Model file for the job. Use its own axes, mm. Coordinates: 2 decimals unless noted, no trailing zeros. Loops run counter-clockwise (first coordinate to the right, second up) from the corner with the lowest first, then second, coordinate; pieces in that order, holes last. Notation, with made-up numbers: (23.25, 24) -> (40.25, 24) arc R9 cw to (40.25, 34) -> close; hole circle Ø2 at (69.25, -17.75). An arc over 180 degrees is marked (long way). Use one line per item in the form item = value.
```python
from build123d import *

# Parameters (mm, degrees)
F0_W     = 609.6
F0_H     = 508
F0_R     = 6.35
F1_DEPTH = 6.35
F2_R     = 3.175
F3_DEPTH = 25.4
F4_R     = 6.35
F5_DEPTH = 25.4
F6_R     = 6.35
F7_DEPTH = 25.4


with BuildPart() as f1:
    # F0 (on Front) → F1 (new body)
    with BuildSketch(Plane.XZ):
        with Locations((304.8, 254)):
            Rectangle(F0_W, F0_H)
        with Locations((279.4, 101.6)):
            Circle(F0_R, mode=Mode.SUBTRACT)
        with Locations((584.2, 101.6)):
            Circle(F0_R, mode=Mode.SUBTRACT)
        with Locations((279.4, 406.4)):
            Circle(F0_R, mode=Mode.SUBTRACT)
        with Locations((584.2, 406.4)):
            Circle(F0_R, mode=Mode.SUBTRACT)
    extrude(amount=F1_DEPTH)

    # F2 (on face) → F3 (cut)
    with BuildSketch(Plane.XZ.offset(6.35)):
        with Locations((209.55, 158.75)):
            Circle(F2_R)
        with Locations((222.25, 158.75)):
            Circle(F2_R)
        with Locations((209.55, 349.25)):
            Circle(F2_R)
        with Locations((222.25, 349.25)):
            Circle(F2_R)
    extrude(amount=-F3_DEPTH, mode=Mode.SUBTRACT)

    # F4 (on face) → F5 (cut)
    with BuildSketch(Plane.XZ.offset(6.35)):
        with Locations((50.8, 406.4)):
            Circle(F4_R)
        with Locations((50.8, 101.6)):
            Circle(F4_R)
    extrude(amount=-F5_DEPTH, mode=Mode.SUBTRACT)

    # F6 (on face) → F7 (cut)
    with BuildSketch(Plane.XZ.offset(6.35)):
        with Locations((203.2, 41.275)):
            Circle(F6_R)
        with Locations((203.2, 466.725)):
            Circle(F6_R)
    extrude(amount=-F7_DEPTH, mode=Mode.SUBTRACT)


solid = f1.part
```
Q1. Mould opens along Z. For faces 1 (the face through (301, 0, 258)), 2 (the face through (54.214, -3.219, 106.954)) say: released by +Z, released by -Z, zero draft, split by the parting line, or undercut.
Result:
face_1 = zero draft
face_2 = undercut
Q2. Band-saw the part on A-A, the plane z = 406.4. Write the cut outline in (x, y).
Result:
outline = (0, -6.35) -> (44.45, -6.35) -> (44.45, 0) -> (0, 0) -> close; (57.15, -6.35) -> (273.05, -6.35) -> (273.05, 0) -> (57.15, 0) -> close; (285.75, -6.35) -> (577.85, -6.35) -> (577.85, 0) -> (285.75, 0) -> close; (590.55, -6.35) -> (609.6, -6.35) -> (609.6, 0) -> (590.55, 0) -> close
Q3. Wall check: line 1 along Z through (x, y) = (51, -5); line 2 along X through (y, z) = (-4.25, 158.75) (3 decimals); line 3 along X through (y, z) = (-1.5, 406.4). Give the ranges that are in metal, low to high.
Result:
line_1 = 0 to 95.25, 107.95 to 400.05, 412.75 to 508
line_2 = 0 to 206.375, 212.725 to 219.075, 225.425 to 609.6
line_3 = 0 to 44.45, 57.15 to 273.05, 285.75 to 577.85, 590.55 to 609.6
